```python
from build123d import *

# Parameters (mm, degrees)
CUT_EXTRUDE1_DEPTH      = 247.268676957
CUT_EXTRUDE1_DEPTH_BACK = 247.268676957


with BuildPart() as part:
    # Sketch2 → Revolve1 (revolve)
    with BuildSketch(Plane(origin=(0, 0, 0), x_dir=(0, 0, -1), z_dir=(1, 0, 0)), mode=Mode.PRIVATE) as revolve1_sk:
        Polygon((-215.9, 9.525), (215.9, 9.525), (222.9, 8.5), (245.9, 8.5), (245.9, 0), (215.9, 0), (215.9, 8.636), (-215.9, 8.636), (-215.9, 0), (-245.9, 0), (-245.9, 8.5), (-222.9, 8.5), align=None)
    revolve(revolve1_sk.sketch.rotate(Axis((0, 0, 215.9), (0, 0, -1)), 90), axis=Axis((0, 0, 215.9), (0, 0, -1)))

    # Sketch3 → Cut-Extrude1 (cut, two sides: drawn at the far end of the back side and taken through both)
    with BuildSketch(Plane(origin=(0, 0, 0), x_dir=(1, 0, 0), z_dir=(0, 1, 0)).offset(-CUT_EXTRUDE1_DEPTH_BACK)):
        Polygon((-7, -220.561998393), (-26.727444109, -220.561998393), (-26.727444109, -252.596471853), (37.522488539, -252.596471853), (37.522488539, -220.561998393), (7, -220.561998393), (7, -245.9), (-7, -245.9), align=None)
        Polygon((-7, 245.9), (-7, 220.561998393), (-26.727444109, 220.561998393), (-26.727444109, 252.596471853), (37.522488539, 252.596471853), (37.522488539, 220.561998393), (7, 220.561998393), (7, 245.9), align=None)
    extrude(amount=CUT_EXTRUDE1_DEPTH + CUT_EXTRUDE1_DEPTH_BACK, mode=Mode.SUBTRACT)


solid = part.part
```
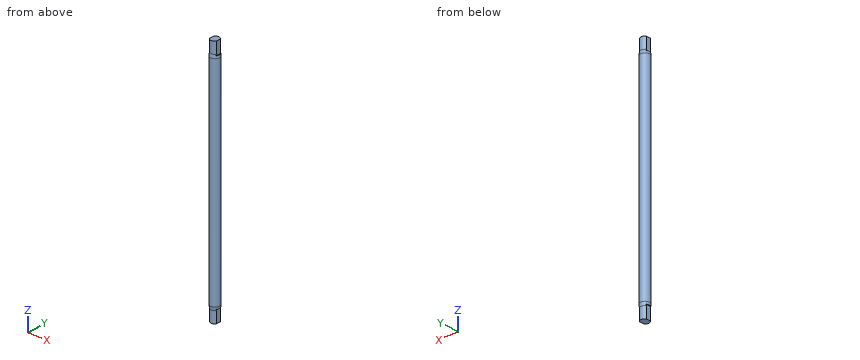
Model file for the job. Use its own axes, mm. Give positions to 0.01 mm unless a question says otherwise; leave off trailing zeros. Write each loop counter-clockwise with the first axis right and the second up, starting at its lowest first coordinate (ties: lowest second). Pieces come first, ordered by that corner, then holes. Notation, with made-up numbers: (24.25, -39) - (53.25, -39) arc R30 cw to (53.25, -6) - close; hole circle Ø1 at (3, 62). An arc over 180 degrees is marked (long way). One line per question, with ' | ' between items. Start each with the question number.
(1) Slice it at A-A on y = 0. Write the cut outline in (x, z) (3 decimals).
(2) Pin check, flat tips, straight feed: P1, Ø5.5, axis at y = 1, z = 239.5, coming from the -X side; P2, Ø4, axis at x = 3.5, z = 86.5, coming from the -Y side; P3, Ø8, axis at x = 5.5, z = -70, coming from the +Y side. Stop position of each tip, or through.
(3) Slice it at C-C on z = 194. Write the cut outline in (x, y) (3 decimals).
(4) Wall check: line 1 along Y through (x, z) = (0, 67) (3 decimals); line 2 along Z through (x, y) = (-8.5, 0.25); line 3 along Z through (x, y) = (-4, 1.5). Give the ranges that are in metal, low to high. Write a range as from..to.
(5) Slice it at B-B on x = 0. Write the cut outline in (y, z) (3 decimals).
Results below:
1) outline: (-9.525, -215.9) - (-8.842, -220.562) - (-7, -220.562) - (-7, -245.9) - (7, -245.9) - (7, -220.562) - (8.842, -220.562) - (9.525, -215.9) - (9.525, 215.9) - (8.842, 220.562) - (7, 220.562) - (7, 245.9) - (-7, 245.9) - (-7, 220.562) - (-8.842, 220.562) - (-9.525, 215.9) - close; hole (-8.636, -215.9) - (8.636, -215.9) - (8.636, 215.9) - (-8.636, 215.9) - close
2) P1: x = -7 | P2: y = -9.41 | P3: y = 9.41
3) outline: circle Ø19.05 at (0, 0); hole circle Ø17.272 at (0, 0)
4) line 1: -9.525..-8.636, 8.636..9.525 | line 2: -220.56..-215.9, 215.9..220.56 | line 3: -245.9..-215.9, 215.9..245.9
5) outline: (-9.525, -215.9) - (-8.5, -222.9) - (-8.5, -245.9) - (8.5, -245.9) - (8.5, -222.9) - (9.525, -215.9) - (9.525, 215.9) - (8.5, 222.9) - (8.5, 245.9) - (-8.5, 245.9) - (-8.5, 222.9) - (-9.525, 215.9) - close; hole (-8.636, -215.9) - (8.636, -215.9) - (8.636, 215.9) - (-8.636, 215.9) - close
